Verification items for this drawing (mm, ordinates from the low corner). A direction names the side the tool comes from. Round coordinates to 2 decimals unless told otherwise and drop trailing zeros. Write each loop counter-clockwise with the first axis right and the second up, starting at its lowest first coordinate (ties: lowest second). Pieces come first, ordered by that corner, then holes.
Item 1: Depth check by flat-ended pin: P1, Ø2, axis at x = 288, y = 586, coming from the +Z side; P2, Ø5, axis at y = 486, z = 271, coming from the -X side; P3, Ø2, axis at x = 222, z = 350, coming from the -Y side. Enter the tip coordinate at first touch or a pass-through.
Item 2: Cross-section at B-B (z = 115). Enter the section's corners in (x, y), then the cut area to 3 significant figures.
Item 3: Cross-section at A-A (x = 249.4). Enter the section's corners in (y, z).
Item 4: Cross-section at C-C (z = 225). Enter the section's corners in (x, y).
Item 5: Access from +Z, -Z, +X, -X, +Y, -Y to the whole of each face (thin tool, end or side, straight path). Record for the marked faces 1, 2 and 3.
Item 6: Cross-section at D-D (y = 73). Enter the section's corners in (x, z), then the cut area to 3 significant figures.
Item 7: Scan lines: probe 1 along Y at (x, z) = (249.4, 161); probe 2 along X at (y, z) = (472, 124); probe 3 along Z at (x, y) = (132.5, 711.5). Record each from-to range of solid material in increasing order.
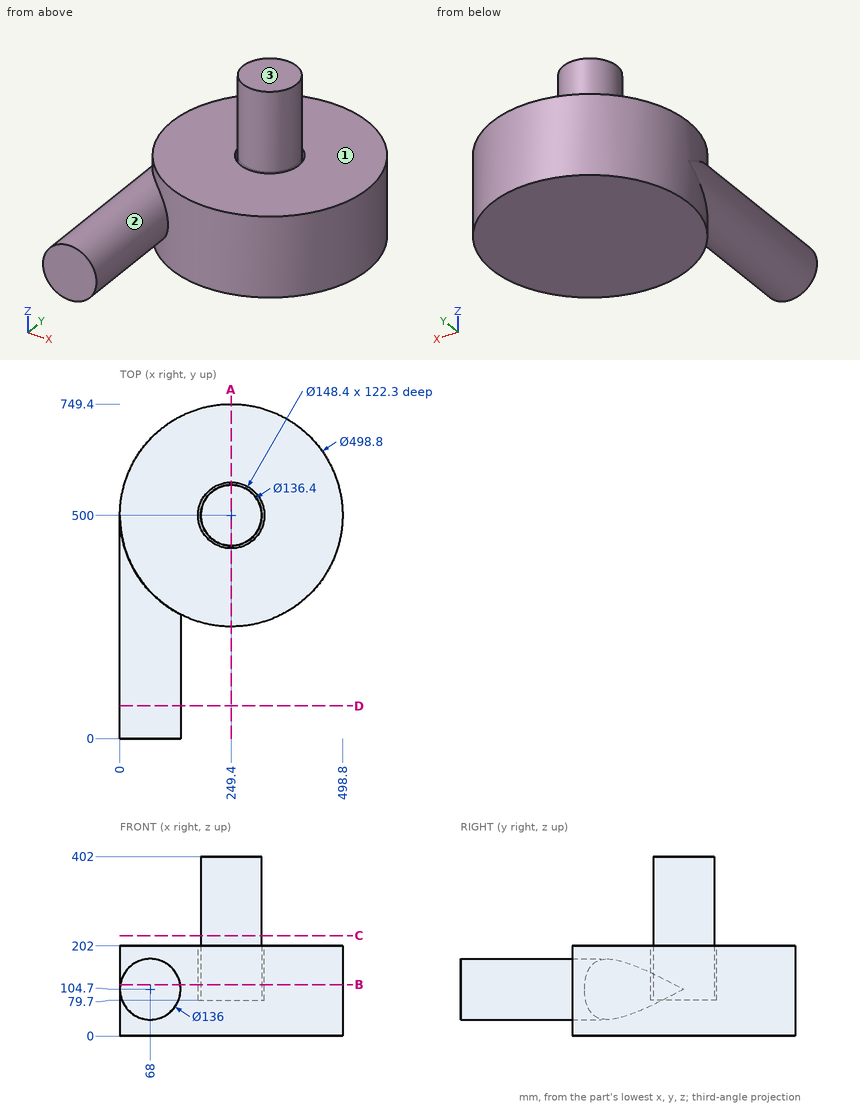
Resolved:
1. P1: stops at z = 202
1. P2: stops at x = 182.18
1. P3: stops at y = 437.12
2. outline: (0.78, 0) - (135.22, 0) - (135.22, 278.27) arc R249.4 ccw (long way) to (0.78, 480.23) - close; circle Ø136.4 at (249.4, 500); hole circle Ø148.4 at (249.4, 500)
2. area: 239,000 mm2
3. outline: (250.6, 0) - (749.4, 0) - (749.4, 202) - (574.2, 202) - (574.2, 79.7) - (568.2, 79.7) - (568.2, 402) - (431.8, 402) - (431.8, 79.7) - (425.8, 79.7) - (425.8, 202) - (250.6, 202) - close
4. outline: circle Ø136.4 at (249.4, 500)
5. face 1: +Z
5. face 2: -Y
5. face 3: +Z, +X, -X, +Y, -Y
6. outline: circle Ø136 at (68, 104.7)
6. area: 14,500 mm2
7. probe 1: y = 250.6 to 425.8, 431.8 to 568.2, 574.2 to 749.4
7. probe 2: x = 1.58 to 180.69, 187.21 to 311.59, 318.11 to 497.22
7. probe 3: z = 0 to 202
